The listing builds one solid part. Answer for the finished solid, in the listing's coordinates (mm). Face numbers are marked on the shaded views. A direction names the side the tool comes from. Coordinates: 2 decimals unless noted, no trailing zeros. Write each loop counter-clockwise with the first axis right and the second up, starting at its lowest first coordinate (ties: lowest second). Pieces come first, ordered by that corner, then holes. Notation, with made-up numbers: M 38.5,3.5 L 73.5,3.5 A20 cw 73.5,35.5 Z; hole C -14,-2 d1. An arc over 180 degrees is marked long. Write item = value, one per line. Start each with the question number.
```python
from build123d import *

# Parameters (mm, degrees)
F0_R             = 80
F1_DEPTH         = 20
F2_R             = 35.8
F3_DEPTH         = 10
F6_R             = 28.55
F7_DEPTH         = 50.001
F9_D             = 15.5
F9_CBORE_D       = 22.25
F9_CBORE_DEPTH   = 14
F9_COPIES_COUNT  = 5
F10_D            = 12.5
F10_COPIES_COUNT = 5
F11_SIZE         = 5
F12_SIZE         = 3


# Not quite as in the source:
# - a pattern or mirror of a feature is missing from the dataset's text; its kind, count and spacing are read off the source's solid
# - the program builds the solid bodies; features that only make, move or delete a surface that nothing else refers to are left out


with BuildPart() as f1:
    # F0 (on Top) → F1 (new body, symmetric)
    with BuildSketch(Plane.XY):
        Circle(F0_R)
    extrude(amount=F1_DEPTH, both=True)

    # F2 (on face) → F3 (join)
    with BuildSketch(Plane.XY.offset(20)):
        Circle(F2_R)
    extrude(amount=F3_DEPTH)

    # F6 (on face) → F7 (cut, through all)
    with BuildSketch(Plane(origin=(0, 0, -20), x_dir=(1, 0, 0), z_dir=(0, 0, -1))):
        Circle(F6_R)
    extrude(amount=-F7_DEPTH, mode=Mode.SUBTRACT)

    # F9 (through all)
    with Locations(Plane.XY.offset(20)):
        with Locations((-30.9016994375, 42.5325404176)):
            f9 = CounterBoreHole(F9_D / 2, F9_CBORE_D / 2, F9_CBORE_DEPTH)

    # F9_copies: F9 ×5 about axis
    f9_copies_axis = Axis((0, 0, 0), (0, 0, 1))
    for i in range(1, F9_COPIES_COUNT):
        add(f9.rotate(f9_copies_axis, i * 360 / F9_COPIES_COUNT), mode=Mode.SUBTRACT)

    # F10 (through all)
    with Locations(Plane.XY.offset(20)):
        with Locations((0, 68.3450445755)):
            f10 = Hole(F10_D / 2)

    # F10_copies: F10 ×5 about axis
    f10_copies_axis = Axis((0, 0, 0), (0, 0, 1))
    for i in range(1, F10_COPIES_COUNT):
        add(f10.rotate(f10_copies_axis, i * 360 / F10_COPIES_COUNT), mode=Mode.SUBTRACT)

    # F11
    f11_edges = [f1.edges().sort_by_distance(p)[0] for p in [
        (-80, 0, 20),
        (-28.55, 0, -20),
        (-80, 0, -20),
    ]]
    chamfer(f11_edges, length=F11_SIZE)

    # F12
    f12_edges = [f1.edges().sort_by_distance(p)[0] for p in [
        (-35.8, 0, 30),
    ]]
    chamfer(f12_edges, length=F12_SIZE)


solid = f1.part
```
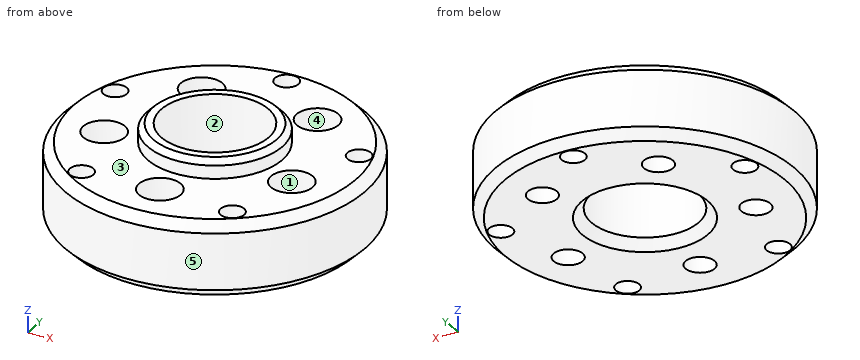
1. For the marked faces 1 and 2, determine the directions among +Z, -Z, +X, -X, +Y, -Y from which every point of the face is accessible in a straight line to the end or side of a thin tool.
2. Straight lines are drawn through the part: L1, parallel to X at y = 45, z = 18.5; L2, parallel to X at y = 41, z = 10; L3, parallel to X at y = -17, z = -15. For each, find the intervals that lie inside material, in ascending order. Write a range as [from, to].
3. For a pull along Y with two mould halves and no side action, classify the marked faces 3, 4 and 5 as pulls with the +Y half, pulls with the -Y half, needs draft (parallel to the pull), parting line crosses it, or undercut.
4. The part is cut by section B-B, the plane x = 0. Count the separate pieces of the cut face and the enclosed holes in it, and give its area (3 significant figures).
5. Each of these flat-tipped pins is pushed along its axis until it touches: pin 1 (18 mm diameter, centred on x = -52, y = -11.5, fed in from +Z); pin 2 (18 mm diameter, centred on x = 50, y = -16.25, fed in from +Z); pin 3 (6 mm diameter, centred on x = 64, y = 56, fed in from -Z); pin 4 (3 mm diameter, centred on y = -25.5, z = 12.5, fed in from +X). Where does it stop, or does it pass through?
6. The part is cut by section A-A, the plane y = 0. Write down the section's boundary in (x, z), and give its area (3 significant figures).
7. The part is cut by section D-D, the plane z = 23.5. Write down the section's boundary in (x, y), and give its area (3 significant figures).
Solution:
q1.face_1 = +Z
q1.face_2 = +Z, -Z
q2.L1 = [-61.86, -41.75], [-20.05, 20.05], [41.75, 61.86]
q2.L2 = [-68.69, -41.92], [-19.88, 19.88], [41.92, 68.69]
q2.L3 = [-78.17, -57.71], [-42.29, -22.94], [22.94, 42.29], [57.71, 78.17]
q3.face_3 = needs draft
q3.face_4 = undercut
q3.face_5 = parting line crosses it
q4.separate_pieces = 4
q4.enclosed_holes = 0
q4.area = 2,960 mm^2
q5.pin_1 = 20
q5.pin_2 = 6
q5.pin_3 = through
q5.pin_4 = 76.32
q6.outline = M -80,-15 L -75,-20 L -33.55,-20 L -28.55,-15 L -28.55,30 L -32.8,30 L -35.8,27 L -35.8,20 L -75,20 L -80,15 Z; M 28.55,-15 L 33.55,-20 L 75,-20 L 80,-15 L 80,15 L 75,20 L 35.8,20 L 35.8,27 L 32.8,30 L 28.55,30 Z
q6.area = 4,180 mm^2
q7.outline = C 0,0 d71.6; hole C 0,0 d57.1
q7.area = 1,470 mm^2
